CAD build for the part. Positions are in the model's coordinates, mm. A direction names the side the tool comes from. Round coordinates to 2 decimals unless told otherwise and drop trailing zeros. Loops run counter-clockwise (first coordinate to the right, second up) from the corner with the lowest first, then second, coordinate; pieces in that order, holes last.
```python
from build123d import *

# Parameters (mm, degrees)
SKETCH_1_R          = 2
EXTRUDE_1_DEPTH     = 7
CUT_EXTRUDE_START   = -5.5
CUT_EXTRUDE_1_DEPTH = 5.5


with BuildPart() as part:
    # 草图1 → 凸台-拉伸1 (new body)
    with BuildSketch(Plane.XY):
        with BuildLine():
            Line((42.5, 0), (60, 0))
            ThreePointArc((60, 0), (15.529142706, 57.955549577), (-51.961524227, 30))
            Line((-51.961524227, 30), (-36.806079661, 21.25))
            ThreePointArc((-36.806079661, 21.25), (10.999809417, 41.051847617), (42.5, 0))
        make_face()
        with Locations((48.219679614, 5.206966288)):
            Circle(SKETCH_1_R, mode=Mode.SUBTRACT)
        with Locations((-37.778343613, 30.41458127)):
            Circle(SKETCH_1_R, mode=Mode.SUBTRACT)
        with Locations((-5.206966288, 48.219679614)):
            Circle(SKETCH_1_R, mode=Mode.SUBTRACT)
        with Locations((30.41458127, 37.778343613)):
            Circle(SKETCH_1_R, mode=Mode.SUBTRACT)
    extrude(amount=EXTRUDE_1_DEPTH)

    # 草图2 → 切除-拉伸1 (cut)
    with BuildSketch(Plane.XY.offset(7).offset(CUT_EXTRUDE_START)):
        with BuildLine():
            Line((52.5, 0), (60, 0))
            ThreePointArc((60, 0), (15.529142706, 57.955549577), (-51.961524227, 30))
            Line((-51.961524227, 30), (-45.466333699, 26.25))
            ThreePointArc((-45.466333699, 26.25), (13.587999868, 50.71110588), (52.5, 0))
        make_face()
    extrude(amount=CUT_EXTRUDE_1_DEPTH, mode=Mode.SUBTRACT)


solid = part.part
```
Item 1: Cut at D-D, the plane y = 14. Give the cut face in (x, z).
Answers follow:
outline: (40.13, 0) - (58.34, 0) - (58.34, 1.5) - (50.6, 1.5) - (50.6, 7) - (40.13, 7) - close
Item 2: Cut at A-A, the plane y = 23.5. Give the cut face in (x, z).
Answers follow:
outline: (-40.7, 0) - (-35.41, 0) - (-35.41, 7) - (-40.7, 7) - close; (35.41, 0) - (55.21, 0) - (55.21, 1.5) - (46.95, 1.5) - (46.95, 7) - (35.41, 7) - close
Item 3: Cut at B-B, the plane z = 5.25. Give the cut face in (x, y), plus the area to 3 significant figures.
Answers follow:
outline: (-45.47, 26.25) - (-36.81, 21.25) arc R42.5 cw to (42.5, 0) - (52.5, 0) arc R52.5 ccw to start; hole circle Ø4 at (-37.78, 30.41); hole circle Ø4 at (-5.21, 48.22); hole circle Ø4 at (30.41, 37.78); hole circle Ø4 at (48.22, 5.21)
area: 1,190 mm2
Item 4: Probe line 1 (Y direction, x = 0.5, z = 4.75); line 2 (X direction, y = 33, z = 0.5); line 3 (Z direction, x = 53, y = 10). List the from-to ranges inside material, lowest first.
Answers follow:
line 1: y = 42.5 to 52.5
line 2: x = -50.11 to -26.78, 26.78 to 50.11
line 3: z = 0 to 1.5
Item 5: Flat gauge pins, fed straight in: P1, Ø3, axis at y = 16.5, z = 4.5, coming from the -X side; P2, Ø4.5, axis at x = -37.78, y = 30.41, coming from the +Z side; P3, Ø2, axis at y = 20, z = 2, coming from the -X side. Where does each tip first touch, or does it go through?
Answers follow:
P1: stops at x = 38.5
P2: stops at z = 7
P3: stops at x = 36.95
Item 6: Two-plate mould, pull along X, no slides. Class faces 1 (the flat face through (11, 42, 7)), 2 (the cylindrical face through (10.246, 41.247, 3.451)), 3 (the flat face through (-42.806, 24.714, 2.673)): released by +X, released by -X, zero draft, split by the parting line, or undercut.
Answers follow:
face 1: zero draft
face 2: undercut
face 3: released by -X
Item 7: 3-axis set-ups, long thin cutter, end or side, ignore diameter. For faces 4 (the cylindrical face through (16.59, 57.66, 0.74)), 5 (the cylindrical face through (12.66, 50.95, 4.21)): which of +Z, -Z, +X, -X, +Y, -Y reach the whole face in a straight line?
Answers follow:
face 4: +Z, -Z, +Y
face 5: +Z, +Y
Item 8: Cut at C-C, the plane x = 21. Give the cut face in (y, z).
Answers follow:
outline: (36.95, 0) - (56.2, 0) - (56.2, 1.5) - (48.12, 1.5) - (48.12, 7) - (36.95, 7) - close
